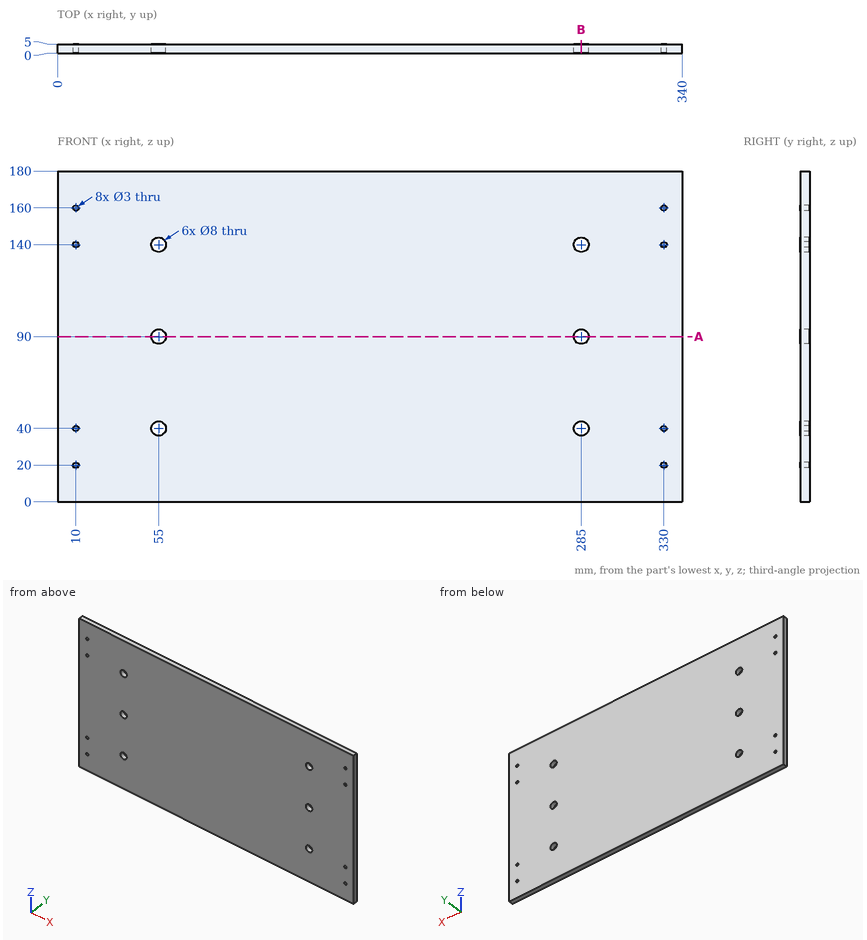
Geometry check sheet. Reference: drawing and pictorial views, mm from the part's lowest x, y, z. Give positions to 0.01 mm unless a question says otherwise; leave off trailing zeros. Write each loop counter-clockwise with the first axis right and the second up, starting at its lowest first coordinate (ties: lowest second). Pieces come first, ordered by that corner, then holes. Notation, with made-up numbers: (86, 59.5) -> (142, 59.5) arc R6 cw to (142, 65.5) -> close; hole circle Ø5 at (18, 82). An arc over 180 degrees is marked (long way). One line per item, written item: value. Start each with the question number.
Item 1: Section check A-A on z = 90. Record the cut outline in (x, y), then the cut area to 3 significant figures.
Item 2: Section check B-B on x = 285. Record the cut outline in (y, z), then the cut area to 3 significant figures.
Item 3: Material ranges on probe 1 along Z at (x, y) = (10, 4); probe 2 along Z at (x, y) = (55, 2.55); probe 3 along X at (y, z) = (4, 140), recorded low to high. Write a range as from..to.
Results list:
1. outline: (0, 0) -> (51, 0) -> (51, 5) -> (0, 5) -> close; (59, 0) -> (281, 0) -> (281, 5) -> (59, 5) -> close; (289, 0) -> (340, 0) -> (340, 5) -> (289, 5) -> close
1. area: 1,620 mm²
2. outline: (0, 0) -> (5, 0) -> (5, 36) -> (0, 36) -> close; (0, 44) -> (5, 44) -> (5, 86) -> (0, 86) -> close; (0, 94) -> (5, 94) -> (5, 136) -> (0, 136) -> close; (0, 144) -> (5, 144) -> (5, 180) -> (0, 180) -> close
2. area: 780 mm²
3. probe 1: 0..18.5, 21.5..38.5, 41.5..138.5, 141.5..158.5, 161.5..180
3. probe 2: 0..36, 44..86, 94..136, 144..180
3. probe 3: 0..8.5, 11.5..51, 59..281, 289..328.5, 331.5..340
